Autodesk Inventor part; units mm, degrees
ref_plane "YZ Plane" through (0, 0, 0) normal (1, 0, 0) x (0, 1, 0)
ref_plane "XZ Plane" through (0, 0, 0) normal (0, 1, 0) x (-1, 0, 0)
ref_plane "XY Plane" through (0, 0, 0) normal (0, 0, 1) x (1, 0, 0)
sketch "Sketch1" plane through (0, 0, 0) normal (0, 0, 1) x (1, 0, 0)
  line L0 (0, 0) -> (300, 0)
  line L1 (0, 0) -> (0, -40)
  line L2 (0, -40) -> (300, -40)
  line L3 (300, -40) -> (300, 0)
  dimension "d0" = 300
  dimension "d1" = 40
extrude "Extrusion1" add sketch "Sketch1" along normal blind 40
sketch "Sketch2" plane through (300, -40, 0) normal (1, 0, 0) x (0, 0, -1)
  line L0 (1, 41) -> (-41, 41)
  line L1 (0, 40) -> (-40, 40)
  line L2 (1, 41) -> (1, -1)
  line L3 (-41, 41) -> (-41, -1)
  line L4 (-41, -1) -> (1, -1)
  line L5 (0, 0) -> (0, 40)
  dimension "d4" = 1
  dimension "d5" = 42
  dimension "d6" = 42
  dimension "d7" = 1
extrude "Extrusion2" add sketch "Sketch2" along normal blind 2
sketch "Sketch3" plane through (0, -40, 0) normal (-1, 0, 0) x (0, 0, 1)
  line L0 (-1, 41) -> (41, 41)
  line L1 (41, 41) -> (41, -1)
  line L2 (41, 41) -> (41, -1)
  line L3 (41, -1) -> (-1, -1)
  line L4 (41, -1) -> (-1, -1)
  line L5 (-1, -1) -> (-1, 41)
  line L6 (-1, -1) -> (-1, 41)
  line L7 (-1, 41) -> (41, 41)
  point P0 (0, 40)
extrude "Extrusion3" add sketch "Sketch3" along normal blind 2
properties part number "InoxLienKet"
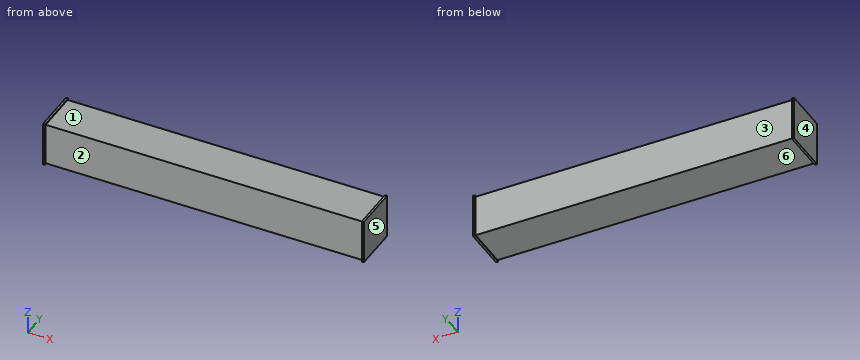
Model file for the job. Use its own axes, mm. Face numbers are marked on the shaded views. A direction names the side the tool comes from. Coordinates: 2 decimals unless noted, no trailing zeros. Write each loop counter-clockwise with the first axis right and the second up, starting at its lowest first coordinate (ties: lowest second). Pieces come first, ordered by that corner, then holes. Notation, with made-up numbers: (73, 50.25) - (127, 50.25) arc R18 cw to (127, 59.25) - close; hole circle Ø9 at (17.5, 39). An arc over 180 degrees is marked (long way). One line per item, written item: value. Start each with the question number.
1. Mould opens along X. For the marked faces 4, 5 and 6 say: released by +X, released by -X, zero draft, split by the parting line, or undercut.
2. Tool access for the marked faces 1, 2 and 3: list every direction of +Z, -Z, +X, -X, +Y, -Y with a clear straight run to the whole face (end or side of a thin tool).
3. Flat gauge pins, fed straight in: pin 1 (12 mm diameter, centred on x = 180, z = 27, fed in from -Y); pin 2 (12 mm diameter, centred on x = 165, y = -12, fed in from -Z); pin 3 (12 mm diameter, centred on x = 160, y = -16.5, fed in from +Z). Where does each tip first touch, or does it go through?
4. Probe line 1 (Z direction, x = 49, y = -34.5); line 2 (Y direction, x = 252, z = 28). List the from-to ranges inside material, lowest first. Write a range as from..to.
5. Slice it at A-A (z = 4.5). Write the cut outline in (x, y).
6. Slice it at B-B (y = -12.5). Write the cut outline in (x, z).
7. Slice it at C-C (x = 68.5). Write the cut outline in (y, z).
Answers below:
1. face 4: released by -X
1. face 5: released by +X
1. face 6: undercut
2. face 1: +Z, +Y, -Y
2. face 2: +Z, -Z, -Y
2. face 3: +Z, -Z, +Y
3. pin 1: stops at y = -40
3. pin 2: stops at z = 0
3. pin 3: stops at z = 40
4. line 1: z = 0..40
4. line 2: y = -40..0
5. outline: (-2, -41) - (0, -41) - (0, -40) - (300, -40) - (300, -41) - (302, -41) - (302, 1) - (300, 1) - (300, 0) - (0, 0) - (0, 1) - (-2, 1) - close
6. outline: (-2, -1) - (0, -1) - (0, 0) - (300, 0) - (300, -1) - (302, -1) - (302, 41) - (300, 41) - (300, 40) - (0, 40) - (0, 41) - (-2, 41) - close
7. outline: (-40, 0) - (0, 0) - (0, 40) - (-40, 40) - close
